Autodesk Inventor part; units mm, degrees
ref_plane "YZ Plane" through (0, 0, 0) normal (1, 0, 0) x (0, 1, 0)
ref_plane "XZ Plane" through (0, 0, 0) normal (0, 1, 0) x (-1, 0, 0)
ref_plane "XY Plane" through (0, 0, 0) normal (0, 0, 1) x (1, 0, 0)
sketch "Sketch1" plane through (0, 0, 0) normal (0, 1, 0) x (-1, 0, 0)
  circle A0 centre (0, 0) radius 18
  line L0 (33.054, 22.5263) -> (-121.3412, 249.0789)
  line L1 (-167, 235) -> (-167, 75.4136)
  circle A1 centre (-142, 235) radius 12.5
  line L2 (0, 0) -> (-142, 0)
  line L3 (33.054, -22.5263) -> (-121.3412, -249.0789)
  line L4 (-167, -235) -> (-167, 75.4136)
  circle A2 centre (-142, -235) radius 12.5
  arc A3 (-121.3412, 249.0789) -> (-167, 235) centre (-142, 235) ccw
  arc A4 (33.054, -22.5263) -> (33.054, 22.5263) centre (0, 0) ccw
  arc A5 (-167, -235) -> (-121.3412, -249.0789) centre (-142, -235) ccw
  point P0 (-167, 316.0765)
  point P1 (-167, -316.0765)
  dimension "d0" = 36
  dimension "d1" = 25
  dimension "d4" = 142
  dimension "d6" = 470
  dimension "d9" = 25
  dimension "d10" = 40
extrude "Extrusion1" add sketch "Sketch1" along normal mid plane 44.45
properties part number "Espacador_Delta"
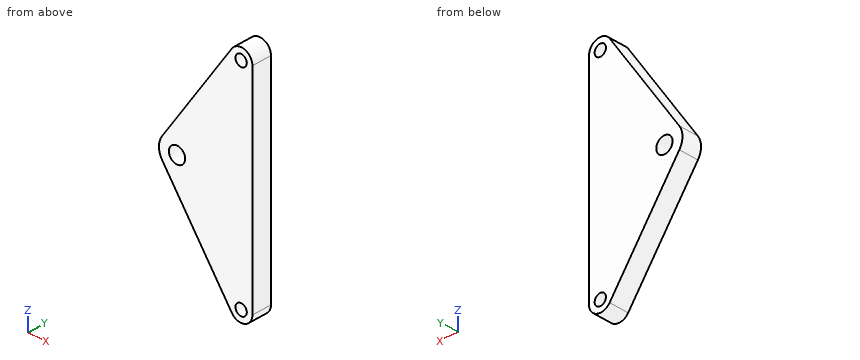
Model file for the job. Use its own axes, mm. Give positions to 0.01 mm unless a question says otherwise; leave off trailing zeros. Order: outer loops, then holes, each group sorted by start corner. A loop starts at its lowest first (then second) coordinate and runs counter-clockwise, first axis right, second up. Notation, with made-up numbers: M 54,36 L 58,36 A13 cw 58,41 Z; hole C 17.25,68 d11. An arc over 180 degrees is marked long. Put each result on its own line as item: value. Start each with the question number.
(1) Band-saw the part on A-A on x = 142. Give the cut face in (y, z) (3 decimals).
(2) Drill centre lines: L1, parallel to Z at x = 142, y = 1.5; L2, parallel to Z at x = 140, y = -7; L3, parallel to Z at x = 10.5, y = -6. Where is each one in solid material? Low to high. Write a range as [from, to].
(3) Band-saw the part on C-C on y = 3.5. Give the cut face in (x, z), then the cut area to 3 significant figures.
(4) Band-saw the part on B-B on z = 0. Give the cut face in (x, y) (3 decimals).
(5) Pin check, flat tips, straight feed: pin 1 Ø1 at (x, y) = (94, 11.5) entering from -Z; pin 2 Ø12 at (x, y) = (-2.5, -17.5) entering from -Z; pin 3 Ø3 at (y, z) = (13.5, -147.5) entering from -X; pin 4 Ø22.5 at (x, z) = (142, 235) entering from -Y. Stop position of each tip, or through.
(6) Band-saw the part on D-D on x = -4.5. Give the cut face in (y, z) (3 decimals), then the cut area to 3 significant figures.
Results below:
1. outline: M -22.225,-260 L 22.225,-260 L 22.225,-247.5 L -22.225,-247.5 Z; M -22.225,-222.5 L 22.225,-222.5 L 22.225,222.5 L -22.225,222.5 Z; M -22.225,247.5 L 22.225,247.5 L 22.225,260 L -22.225,260 Z
2. L1: z = [-260, -247.5], [-222.5, 222.5], [247.5, 260]
2. L2: z = [-259.92, -247.34], [-222.66, 222.66], [247.34, 259.92]
2. L3: z = [-86.44, -14.62], [14.62, 86.44]
3. outline: M -33.05,-22.53 L 121.34,-249.08 A25 ccw 167,-235 L 167,235 A25 ccw 121.34,249.08 L -33.05,22.53 A40 ccw Z; hole C 0,0 d36; hole C 142,-235 d25; hole C 142,235 d25
3. area: 63,500 mm2
4. outline: M -40,-22.225 L -18,-22.225 L -18,22.225 L -40,22.225 Z; M 18,-22.225 L 167,-22.225 L 167,22.225 L 18,22.225 Z
5. pin 1: stops at z = -209.69
5. pin 2: stops at z = -76.16
5. pin 3: stops at x = 51.09
5. pin 4: passes through
6. outline: M -22.225,-64.425 L 22.225,-64.425 L 22.225,-17.428 L -22.225,-17.428 Z; M -22.225,17.428 L 22.225,17.428 L 22.225,64.425 L -22.225,64.425 Z
6. area: 4,180 mm2
